Read the model definition and answer for the solid it produces. Units are mm, in the model's axes. Face numbers are marked on the shaded views. A direction names the side the tool comes from. Coordinates: 2 decimals unless noted, no trailing zeros. Loops run counter-clockwise (first coordinate to the right, second up) from the corner with the lowest first, then second, coordinate; pieces in that order, holes last. Notation, with made-up numbers: (-39, -23.5) -> (-28, -23.5) arc R16 ccw to (-28, -1.5) -> close; hole circle Ø8 at (23, 52.25). An arc over 180 degrees is marked (long way). Answer in a Markdown table with one row per item.
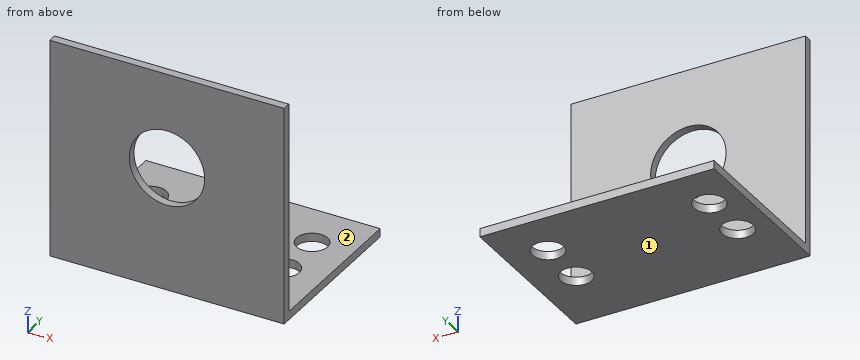
```python
from build123d import *

# Parameters (mm, degrees)
SKETCH_W                        = 45
SKETCH_H                        = 42
PAD_DEPTH                       = 1.6
SKETCH001_W                     = 45
SKETCH001_H                     = 1.6
PAD001_DEPTH                    = 31
SKETCH002_R                     = 7.25
POCKET_DEPTH                    = 32.601
SKETCH003_R                     = 3
POCKET001_DEPTH                 = 140.910153
SKETCH003_LINEARPATTERN_2_R     = 3
POCKET001_LINEARPATTERN_2_DEPTH = 140.910153
LINEARPATTERN001_COUNT          = 2
LINEARPATTERN001_PITCH          = 31


with BuildPart() as part:
    # Sketch → Pad (new body)
    with BuildSketch(Plane.XZ):
        with Locations((22.5, 21)):
            Rectangle(SKETCH_W, SKETCH_H)
    extrude(amount=PAD_DEPTH)

    # Sketch001 (on Face5 of Pad) → Pad001 (join)
    with BuildSketch(Plane(origin=(0, 0, 0), x_dir=(1, 0, 0), z_dir=(0, 1, 0))):
        with Locations((22.5, -0.8)):
            Rectangle(SKETCH001_W, SKETCH001_H)
    extrude(amount=PAD001_DEPTH)

    # Sketch002 (on Face5 of Pad001) → Pocket (cut, through all)
    with BuildSketch(Plane.XZ.offset(1.6)):
        with Locations((22.5, 23.75)):
            Circle(SKETCH002_R)
    extrude(amount=-POCKET_DEPTH, mode=Mode.SUBTRACT)

    # Sketch003 (on Face12 of Pocket) → Pocket001 (cut, through all)
    with BuildSketch(Plane(origin=(0, 0, 1.6), x_dir=(-1, 0, 0), z_dir=(0, 0, 1))):
        with Locations((-6.3, -11.9)):
            Circle(SKETCH003_R)
    pocket001 = extrude(amount=-POCKET001_DEPTH, mode=Mode.SUBTRACT)

    # Sketch003 LinearPattern 2 → Pocket001 LinearPattern 2 (cut, through all)
    with BuildSketch(Plane(origin=(0, 9.6, 1.6), x_dir=(-1, 0, 0), z_dir=(0, 0, 1))):
        with Locations((-6.3, -11.9)):
            Circle(SKETCH003_LINEARPATTERN_2_R)
    pocket001_linearpattern_2 = extrude(amount=-POCKET001_LINEARPATTERN_2_DEPTH, mode=Mode.SUBTRACT)

    # LinearPattern001: Pocket001, Pocket001 LinearPattern 2 ×2
    with Locations(*[(i * LINEARPATTERN001_PITCH, 0, 0) for i in range(1, LINEARPATTERN001_COUNT)]):
        add(pocket001, mode=Mode.SUBTRACT)
        add(pocket001_linearpattern_2, mode=Mode.SUBTRACT)


solid = part.part
```
1. A cutting plane is placed at A-A on y = 11.9. Give the vertices of the cut face in (x, z), and give its area (3 significant figures).
A:
| item | result |
|---|---|
| outline | (0, 0) -> (3.3, 0) -> (3.3, 1.6) -> (0, 1.6) -> close; (9.3, 0) -> (34.3, 0) -> (34.3, 1.6) -> (9.3, 1.6) -> close; (40.3, 0) -> (45, 0) -> (45, 1.6) -> (40.3, 1.6) -> close |
| area | 52.8 mm2 |
2. Find the intervals of material crossed by probe 1 along X at (y, z) = (21.5, 0.6); probe 2 along Y at (x, z) = (6.3, 0.65); probe 3 along Z at (x, y) = (22.5, -0.4), in increasing order.
A:
| item | result |
|---|---|
| probe 1 | x = 0 to 3.3, 9.3 to 34.3, 40.3 to 45 |
| probe 2 | y = -1.6 to 8.9, 14.9 to 18.5, 24.5 to 31 |
| probe 3 | z = 0 to 16.5, 31 to 42 |
3. A cutting plane is placed at C-C on z = 23.75. Give the vertices of the cut face in (x, y).
A:
| item | result |
|---|---|
| outline | (0, -1.6) -> (15.25, -1.6) -> (15.25, 0) -> (0, 0) -> close; (29.75, -1.6) -> (45, -1.6) -> (45, 0) -> (29.75, 0) -> close |
4. Given pin 1 Ø8 at (x, z) = (39.5, 33) entering from +Y; pin 2 Ø3.5 at (x, y) = (37.3, 21.5) entering from -Z; pin 3 Ø6 at (x, y) = (13.5, 26.5) entering from +Z, each flat-ended and moving along its own axis, determine where each tip first touches the part or whether it passes through.
A:
| item | result |
|---|---|
| pin 1 | stops at y = 0 |
| pin 2 | passes through |
| pin 3 | stops at z = 1.6 |
5. A cutting plane is placed at B-B on x = 22.5. Give the vertices of the cut face in (y, z).
A:
| item | result |
|---|---|
| outline | (-1.6, 0) -> (31, 0) -> (31, 1.6) -> (0, 1.6) -> (0, 16.5) -> (-1.6, 16.5) -> close; (-1.6, 31) -> (0, 31) -> (0, 42) -> (-1.6, 42) -> close |
6. A cutting plane is placed at D-D on x = 6.3. Give the vertices of the cut face in (y, z).
A:
| item | result |
|---|---|
| outline | (-1.6, 0) -> (8.9, 0) -> (8.9, 1.6) -> (0, 1.6) -> (0, 42) -> (-1.6, 42) -> close; (14.9, 0) -> (18.5, 0) -> (18.5, 1.6) -> (14.9, 1.6) -> close; (24.5, 0) -> (31, 0) -> (31, 1.6) -> (24.5, 1.6) -> close |
7. A tool of negligible diameter and unlimited length cuts with its end or side. For the marked faces 1 and 2, from which of +Z, -Z, +X, -X, +Y, -Y can it reach the whole face along a straight path? Write none if from no direction.
A:
| item | result |
|---|---|
| face 1 | -Z, +X, -X, +Y, -Y |
| face 2 | +Z, +X, -X, +Y |
